Part model, mm, in its own coordinate system. A direction names the side the tool comes from. Give positions to 0.01 mm unless a question says otherwise; leave off trailing zeros. Write each loop counter-clockwise with the first axis right and the second up, starting at its lowest first coordinate (ties: lowest second). Pieces come first, ordered by that corner, then holes.
```python
from build123d import *

# Parameters (mm, degrees)
BOSS_EXTRUDE1_DEPTH = 12.7
FILLET1_R           = 1.5
FILLET2_R           = 1.5
SKETCH4_R           = 1.85
CUT_EXTRUDE1_DEPTH  = 63.498108771
SKETCH11_W          = 12
SKETCH11_H          = 25
CUT_EXTRUDE2_DEPTH  = 12.7


with BuildPart() as part:
    # Sketch1 → Boss-Extrude1 (new body)
    with BuildSketch(Plane.XY):
        Polygon((11.25, -11.44), (26.25, -11.44), (26.25, 31.44), (-26.25, 31.44), (-26.25, -11.44), (-11.25, -11.44), (-11.25, -3.56), (11.25, -3.56), align=None)
    extrude(amount=BOSS_EXTRUDE1_DEPTH)

    # Fillet1
    fillet1_edges = [part.edges().sort_by_distance(p)[0] for p in [
        (-26.25, 31.44, 6.35),
    ]]
    fillet(fillet1_edges, radius=FILLET1_R)

    # Fillet2
    fillet2_edges = [part.edges().sort_by_distance(p)[0] for p in [
        (-11.25, -3.56, 6.35),
    ]]
    fillet(fillet2_edges, radius=FILLET2_R)

    # Sketch4 → Cut-Extrude1 (cut, through all)
    with BuildSketch(Plane.ZY.offset(26.25)):
        with Locations(Location((6.35, -7.56, 0), (0, 0, 270))):
            Circle(SKETCH4_R)
    extrude(amount=-CUT_EXTRUDE1_DEPTH, mode=Mode.SUBTRACT)

    # Sketch11 → Cut-Extrude2 (cut)
    with BuildSketch(Plane.XY.offset(12.7)):
        with Locations((5.25, 13.945)):
            Rectangle(SKETCH11_W, SKETCH11_H)
    extrude(amount=-CUT_EXTRUDE2_DEPTH, mode=Mode.SUBTRACT)


solid = part.part
```
1) Wall check: L1, parallel to X at y = -9, z = 5; L2, parallel to X at y = 23, z = 7; L3, parallel to Z at x = -23, y = -7.56. Give the ranges that are in metal, low to high.
Answers follow:
L1: x = -26.25 to -11.25, 11.25 to 26.25
L2: x = -26.25 to -0.75, 11.25 to 26.25
L3: z = 0 to 4.5, 8.2 to 12.7
2) Saw through at A-A, the plane z = 6.35. Write the cut outline in (x, y) (3 decimals), then the cut area to 3 significant figures.
Answers follow:
outline: (-26.25, -11.44) - (-11.25, -11.44) - (-11.25, -9.41) - (-26.25, -9.41) - close; (-26.25, -5.71) - (-11.25, -5.71) - (-11.25, -5.06) arc R1.5 cw to (-9.75, -3.56) - (11.25, -3.56) - (11.25, -5.71) - (26.25, -5.71) - (26.25, 31.44) - (-24.75, 31.44) arc R1.5 ccw to (-26.25, 29.94) - close; (11.25, -11.44) - (26.25, -11.44) - (26.25, -9.41) - (11.25, -9.41) - close; hole (-0.75, 1.445) - (11.25, 1.445) - (11.25, 26.445) - (-0.75, 26.445) - close
area: 1,660 mm2
3) Two-plate mould, pull along X, no slides. Class faces 4 (the face through (5, 1.445, 6)), 5 (the face through (-0.75, 14, 6)), 6 (the face through (-26.25, 10, 6)), 7 (the face through (18.645, -6.196, 7.6)): +X half, -X half, draft (parallel to the pull), parting line (faces both ways), or undercut.
Answers follow:
face 4: undercut
face 5: undercut
face 6: -X half
face 7: draft
4) Saw through at B-B, the plane y = -7.56. Write the cut outline in (x, z).
Answers follow:
outline: (-26.25, 0) - (-11.25, 0) - (-11.25, 4.5) - (-26.25, 4.5) - close; (-26.25, 8.2) - (-11.25, 8.2) - (-11.25, 12.7) - (-26.25, 12.7) - close; (11.25, 0) - (26.25, 0) - (26.25, 4.5) - (11.25, 4.5) - close; (11.25, 8.2) - (26.25, 8.2) - (26.25, 12.7) - (11.25, 12.7) - close
5) Saw through at C-C, the plane x = 6. Write the cut outline in (y, z) (3 decimals), then the cut area to 3 significant figures.
Answers follow:
outline: (-3.56, 0) - (1.445, 0) - (1.445, 12.7) - (-3.56, 12.7) - close; (26.445, 0) - (31.44, 0) - (31.44, 12.7) - (26.445, 12.7) - close
area: 127 mm2
6) Pin check, flat tips, straight feed: pin 1 Ø2 at (y, z) = (-7.56, 6.35) entering from +X; pin 2 Ø3.5 at (x, z) = (3, 6) entering from -Y. Stop position of each tip, or through.
Answers follow:
pin 1: passes through
pin 2: stops at y = -3.56
7) 3-axis set-ups, long thin cutter, end or side, ignore diameter. For faces 1 (the face through (11.25, -6, 8)), 2 (the face through (19, -11.44, 6)), 3 (the face through (11.25, 14, 6)): which of +Z, -Z, +X, -X, +Y, -Y reach the whole face in a straight line?
Answers follow:
face 1: +Z, -Z, -Y
face 2: +Z, -Z, +X, -X, -Y
face 3: +Z, -Z
8) Saw through at D-D, the plane y = 7.5. Write the cut outline in (x, z).
Answers follow:
outline: (-26.25, 0) - (-0.75, 0) - (-0.75, 12.7) - (-26.25, 12.7) - close; (11.25, 0) - (26.25, 0) - (26.25, 12.7) - (11.25, 12.7) - close
